Verification items for the finished model (mm, model axes). Give positions to 0.01 mm unless a question says otherwise; leave off trailing zeros. Loops run counter-clockwise (first coordinate to the right, second up) from the corner with the lowest first, then second, coordinate; pieces in that order, holes last. Notation, with made-up numbers: M 56.5,-11.5 L 106.5,-11.5 A32 cw 106.5,19.5 Z; hole C 89.25,-37 d4. An arc over 180 degrees is marked long. Put each result on its own line as item: value. Start each with the question number.
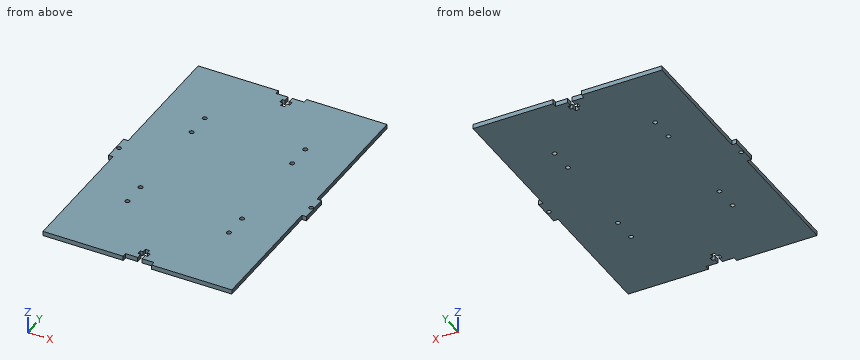
from build123d import *

# Parameters (mm, degrees)
SKETCH1_W           = 139.7
SKETCH1_H           = 203.2
BOSS_EXTRUDE1_DEPTH = 3.18
SKETCH2_R           = 1.5
SKETCH2_W           = 3.18
SKETCH2_H           = 91.725
CUT_EXTRUDE1_DEPTH  = 4.18
SKETCH3_R           = 1.59
CUT_EXTRUDE2_DEPTH  = 4.18
SKETCH4_R           = 1.59
CUT_EXTRUDE3_DEPTH  = 4.18


with BuildPart() as part:
    # Sketch1 → Boss-Extrude1 (new body)
    with BuildSketch(Plane.XY):
        Rectangle(SKETCH1_W, SKETCH1_H)
    extrude(amount=BOSS_EXTRUDE1_DEPTH)

    # Sketch2 → Cut-Extrude1 (cut, through all)
    with BuildSketch(Plane.XY.offset(3.18)):
        with Locations((-67.85, 0)):
            Circle(SKETCH2_R)
        with Locations((67.85, 0)):
            Circle(SKETCH2_R)
        Polygon((-10, 101.6), (10, 101.6), (10, 98.42), (1.5, 98.42), (1.5, 94.42), (3.5, 94.42), (3.5, 91.42), (1.5, 91.42), (1.5, 88.42), (-1.5, 88.42), (-1.5, 91.42), (-3.5, 91.42), (-3.5, 94.42), (-1.5, 94.42), (-1.5, 98.42), (-10, 98.42), align=None)
        Polygon((-10, -101.6), (-10, -98.42), (-1.5, -98.42), (-1.5, -94.42), (-3.5, -94.42), (-3.5, -91.42), (-1.5, -91.42), (-1.5, -88.42), (1.5, -88.42), (1.5, -91.42), (3.5, -91.42), (3.5, -94.42), (1.5, -94.42), (1.5, -98.42), (10, -98.42), (10, -101.6), align=None)
        with Locations((-68.26, 55.7375)):
            Rectangle(SKETCH2_W, SKETCH2_H)
        with Locations((-68.26, -55.7375)):
            Rectangle(SKETCH2_W, SKETCH2_H)
        with Locations((68.26, -55.7375)):
            Rectangle(SKETCH2_W, SKETCH2_H)
        with Locations((68.26, 55.7375)):
            Rectangle(SKETCH2_W, SKETCH2_H)
    extrude(amount=-CUT_EXTRUDE1_DEPTH, mode=Mode.SUBTRACT)

    # Sketch3 → Cut-Extrude2 (cut, through all)
    with BuildSketch(Plane(origin=(0, 0, 0), x_dir=(-1, 0, 0), z_dir=(0, 0, -1))):
        with Locations((-35.67127699, -47.963396943)):
            Circle(SKETCH3_R)
        with Locations((-35.67127699, -30.777287406)):
            Circle(SKETCH3_R)
    extrude(amount=-CUT_EXTRUDE2_DEPTH, mode=Mode.SUBTRACT)

    # Sketch4 → Cut-Extrude3 (cut, through all)
    with BuildSketch(Plane(origin=(0, 0, 0), x_dir=(-1, 0, 0), z_dir=(0, 0, -1))):
        with Locations((-34.750723073, 53.780323187)):
            Circle(SKETCH4_R)
        with Locations((-34.750723073, 36.59421365)):
            Circle(SKETCH4_R)
        with Locations((36.249784221, 53.780323187)):
            Circle(SKETCH4_R)
        with Locations((36.249784221, 36.59421365)):
            Circle(SKETCH4_R)
        with Locations((35.983928162, -30.777287406)):
            Circle(SKETCH4_R)
        with Locations((35.983928162, -47.963396943)):
            Circle(SKETCH4_R)
        with Locations((-35.67127699, -30.777287406)):
            Circle(SKETCH4_R)
        with Locations((-35.67127699, -47.963396943)):
            Circle(SKETCH4_R)
    extrude(amount=-CUT_EXTRUDE3_DEPTH, mode=Mode.SUBTRACT)


solid = part.part
Q1. Scan lines: L1, parallel to X at y = 93, z = 0.6; L2, parallel to X at y = -89, z = 0.45; L3, parallel to Y at x = -67.85, z = 2 (3 decimals). Record each from-to range of solid material in increasing order.
Q2. Cross-section at B-B, the plane z = 2.45. State how many separate pieces and enclosed holes the cut face has, then the cut area to 3 significant figures.
Q3. Cross-section at A-A, the plane y = -79.5. Record the boundary of the cut face in (x, z), then the cut area to 3 significant figures.
Q4. Go/stop test with flat-tipped pins: pin 1 (1 mm diameter, centred on x = 68.5, z = 2, fed in from -Y) (3 decimals); pin 2 (1.5 mm diameter, centred on y = -50.5, z = 1, fed in from +X); pin 3 (1.6 mm diameter, centred on x = 3, z = 1, fed in from +Y); pin 4 (3 mm diameter, centred on x = -36.25, y = 53.78, fed in from -Z). Record where each tip stops, or that it passes through.
Ans:
1. L1: x = -66.67 to -3.5, 3.5 to 66.67
1. L2: x = -66.67 to -1.5, 1.5 to 66.67
1. L3: y = -9.875 to -1.5, 1.5 to 9.875
2. separate pieces: 1
2. enclosed holes: 10
2. area: 26,900 mm^2
3. outline: M -66.67,0 L 66.67,0 L 66.67,3.18 L -66.67,3.18 Z
3. area: 424 mm^2
4. pin 1: stops at y = -9.875
4. pin 2: stops at x = 66.67
4. pin 3: stops at y = 98.42
4. pin 4: passes through
